Input: part model. Units: mm. Frame: model coordinates. A direction names the side the tool comes from. Give positions to 0.01 mm unless a question says otherwise; leave off trailing zeros. Write each loop counter-clockwise with the first axis right and the second up, starting at its lowest first coordinate (ties: lowest second). Pieces come first, ordered by that corner, then holes. Notation, with made-up numbers: (48.5, -37) -> (64.5, -37) arc R20 cw to (64.5, -30) -> close; hole circle Ø6 at (-3, 59). An arc over 180 degrees is marked (long way). Answer as a JSON object with one key per item and string values. Group by question number.
from build123d import *

# Parameters (mm, degrees)
F0_R     = 8.5
F0_W     = 304.8
F0_H     = 304.8
F1_DEPTH = 15.5


with BuildPart() as f1:
    # F0 (on Front) → F1 (new body)
    with BuildSketch(Plane.XZ):
        with BuildLine():
            ThreePointArc((-306.680941, 234.30534), (-313.752009, 231.376408), (-316.680941, 224.30534))
            Line((-316.680941, 224.30534), (-316.680941, -163.899746))
            ThreePointArc((-316.680941, -163.899746), (-314.280706, -169.694425), (-308.486027, -172.09466))
            Line((-308.486027, -172.09466), (79.719059, -172.09466))
            ThreePointArc((79.719059, -172.09466), (86.790127, -169.165728), (89.719059, -162.09466))
            Line((89.719059, -162.09466), (89.719059, 224.30534))
            ThreePointArc((89.719059, 224.30534), (86.790127, 231.376408), (79.719059, 234.30534))
            Line((79.719059, 234.30534), (-306.680941, 234.30534))
        make_face()
        with Locations((-296.680941, -152.09466)):
            Circle(F0_R, mode=Mode.SUBTRACT)
        with Locations((-174.547941, -152.09466)):
            Circle(F0_R, mode=Mode.SUBTRACT)
        with Locations((-296.680941, -29.96166)):
            Circle(F0_R, mode=Mode.SUBTRACT)
        with Locations((-52.414941, -152.09466)):
            Circle(F0_R, mode=Mode.SUBTRACT)
        with Locations((69.719059, -152.09466)):
            Circle(F0_R, mode=Mode.SUBTRACT)
        with Locations((-113.480941, 31.10534)):
            Rectangle(F0_W, F0_H, mode=Mode.SUBTRACT)
        with Locations((69.719059, -29.96166)):
            Circle(F0_R, mode=Mode.SUBTRACT)
        with Locations((-296.680941, 92.17134)):
            Circle(F0_R, mode=Mode.SUBTRACT)
        with Locations((-296.680941, 214.30534)):
            Circle(F0_R, mode=Mode.SUBTRACT)
        with Locations((-174.546941, 214.30534)):
            Circle(F0_R, mode=Mode.SUBTRACT)
        with Locations((69.719059, 92.17134)):
            Circle(F0_R, mode=Mode.SUBTRACT)
        with Locations((-52.413941, 214.30534)):
            Circle(F0_R, mode=Mode.SUBTRACT)
        with Locations((69.719059, 214.30434)):
            Circle(F0_R, mode=Mode.SUBTRACT)
    extrude(amount=F1_DEPTH)


solid = f1.part
1. Line query: line 1 (Z direction, x = -52.5, y = -10.5); line 2 (Z direction, x = -194.5, y = -1.75); line 3 (Z direction, x = 65.5, y = -5.75). Output: solid intervals per line, ascending.
2. Section A-A (x = -121.5). Return the cut outline in (y, z), plus the area to 3 significant figures.
3. Section B-B (z = 152.5). Return the cut outline in (x, y).
4. Reachability of faces 4 (the face through (-316.681, -8, 33)), 5 (the face through (38.919, -8, 29)) from +Z, -Z, +X, -X, +Y, -Y: full face, straight path, thin tool, end or side. Return the list, or none.
5. Contact query for a flat-ended pin moving along its axis: pin 1 Ø22 at (x, z) = (-52.41, -152.09) entering from +Y. Output: stop coordinate, or through.
6. Mould query, pull axis Z, two halves, no side actions, for faces 1 (the face through (-280, 0, 47)), 2 (the face through (-111, -8, 234.305)), 3 (the face through (63.454, -7.642, 220.049)). Classes: pulls with the +Z half, pulls with the -Z half, needs draft (parallel to the pull), parting line crosses it, or undercut.
7. Section C-C (y = -5.25). State how many separate pieces and enclosed holes the cut face has, plus the area to 3 significant figures.
Working result:
{
 "1": {"line 1": "z = -172.09 to -160.59, -143.6 to -121.29, 183.51 to 205.81, 222.8 to 234.31", "line 2": "z = -172.09 to -121.29, 183.51 to 234.31", "line 3": "z = -172.09 to -159.47, -144.72 to -37.34, -22.58 to 84.79, 99.55 to 206.93, 221.68 to 234.31"},
 "2": {"outline": "(-15.5, -172.09) -> (0, -172.09) -> (0, -121.29) -> (-15.5, -121.29) -> close; (-15.5, 183.51) -> (0, 183.51) -> (0, 234.31) -> (-15.5, 234.31) -> close", "area": "1,570 mm^2"},
 "3": {"outline": "(-316.68, -15.5) -> (-265.88, -15.5) -> (-265.88, 0) -> (-316.68, 0) -> close; (38.92, -15.5) -> (89.72, -15.5) -> (89.72, 0) -> (38.92, 0) -> close"},
 "4": {"face 4": "+Z, -Z, -X, +Y, -Y", "face 5": "+Y, -Y"},
 "5": {"pin 1": "stops at y = 0"},
 "6": {"face 1": "needs draft", "face 2": "pulls with the +Z half", "face 3": "undercut"},
 "7": {"separate pieces": "1", "enclosed holes": "13", "area": "69,500 mm^2"}
}
